```python
from build123d import *

# Parameters (mm, degrees)
SKETCH1_W      = 22
SKETCH1_H      = 12
EXTRUDE1_DEPTH = 10
SKETCH2_W      = 30
SKETCH2_H      = 12
EXTRUDE2_DEPTH = 2
SKETCH3_W      = 22
SKETCH3_H      = 12
EXTRUDE3_DEPTH = 4
SKETCH4_R      = 1
EXTRUDE4_DEPTH = 13
EXTRUDE5_DEPTH = 3.8
SKETCH6_R      = 2.25
EXTRUDE6_DEPTH = 4


with BuildPart() as part:
    # Sketch1 → Extrude1 (new body)
    with BuildSketch(Plane.XY):
        Rectangle(SKETCH1_W, SKETCH1_H)
    extrude(amount=EXTRUDE1_DEPTH)

    # Sketch2 → Extrude2 (add)
    with BuildSketch(Plane.XY.offset(10)):
        Rectangle(SKETCH2_W, SKETCH2_H)
    extrude(amount=EXTRUDE2_DEPTH)

    # Sketch3 → Extrude3 (add)
    with BuildSketch(Plane.XY.offset(12)):
        Rectangle(SKETCH3_W, SKETCH3_H)
    extrude(amount=EXTRUDE3_DEPTH)

    # Sketch4 → Extrude4 (cut, through all)
    with BuildSketch(Plane.XY.offset(12)):
        with Locations((-13, 0)):
            Circle(SKETCH4_R)
        with Locations((13, 0)):
            Circle(SKETCH4_R)
    extrude(amount=-EXTRUDE4_DEPTH, mode=Mode.SUBTRACT)

    # Sketch5 → Extrude5 (add)
    with BuildSketch(Plane.XY.offset(16)):
        with BuildLine():
            ThreePointArc((-0.479166667, -2.445144707), (11, 0), (-0.479166667, 2.445144707))
            ThreePointArc((-0.479166667, 2.445144707), (-3.5, 0), (-0.479166667, -2.445144707))
        make_face()
    extrude(amount=EXTRUDE5_DEPTH)

    # Sketch6 → Extrude6 (add)
    with BuildSketch(Plane.XY.offset(19.8)):
        with Locations((5, 0)):
            Circle(SKETCH6_R)
    extrude(amount=EXTRUDE6_DEPTH)


solid = part.part
```
CAD build for the part. Positions are in the model's coordinates, mm. A direction names the side the tool comes from. Give positions to 0.01 mm unless a question says otherwise; leave off trailing zeros. Order: outer loops, then holes, each group sorted by start corner. A loop starts at its lowest first (then second) coordinate and runs counter-clockwise, first axis right, second up.
(1) Saw through at B-B, the plane x = -1. Give the cut face in (y, z).
(2) Flat gauge pins, fed straight in: pin 1 (2.5 mm diameter, centred on x = 13, y = 0, fed in from +Z); pin 2 (5 mm diameter, centred on y = 0.5, z = 6.5, fed in from -X); pin 3 (1.2 mm diameter, centred on x = -12, y = 1, fed in from -Z); pin 4 (1.2 mm diameter, centred on x = -13, y = 0, fed in from -Z). Where does each tip first touch, or does it go through?
(3) Saw through at C-C, the plane z = 20.75. Give the cut face in (x, y).
(4) Mould opens along X. For faces 5 (the cylindrical face through (7.146, 0.676, 21.772)), 6 (the cylindrical face through (-12, 0, 11)), 7 (the flat face through (11, 0, 5)), 8 (the flat face through (10, 5, 16)) say: released by +X, released by -X, zero draft, split by the parting line, or undercut.
(5) Drill centre lines: L1, parallel to Y at x = -13, z = 11.1; L2, parallel to X at y = 5, z = 13.25; L3, parallel to Z at x = -2.5, y = -3.25. Where is each one in solid material? Low to high.
(6) Saw through at A-A, the plane x = 13. Give the cut face in (y, z).
(7) Saw through at D-D, the plane y = -3. Give the cut face in (x, z).
(8) Tool access for faces 1 (the flat face through (-11.7, 0.1, 12)), 2 (the flat face through (10, -5, 16)), 3 (the flat face through (14.3, 0.1, 10)), 4 (the flat face through (-11.7, 0.1, 10)): list every direction of +Z, -Z, +X, -X, +Y, -Y with a clear straight run to the whole face (end or side of a thin tool).
Results found:
1. outline: (-6, 0) - (6, 0) - (6, 16) - (2.5, 16) - (2.5, 19.8) - (-2.5, 19.8) - (-2.5, 16) - (-6, 16) - close
2. pin 1: stops at z = 12
2. pin 2: stops at x = -11
2. pin 3: stops at z = 10
2. pin 4: passes through
3. outline: circle Ø4.5 at (5, 0)
4. face 5: split by the parting line
4. face 6: undercut
4. face 7: released by +X
4. face 8: zero draft
5. L1: y = -6 to -1, 1 to 6
5. L2: x = -11 to 11
5. L3: z = 0 to 16
6. outline: (-6, 10) - (-1, 10) - (-1, 12) - (-6, 12) - close; (1, 10) - (6, 10) - (6, 12) - (1, 12) - close
7. outline: (-15, 10) - (-11, 10) - (-11, 0) - (11, 0) - (11, 10) - (15, 10) - (15, 12) - (11, 12) - (11, 16) - (10.2, 16) - (10.2, 19.8) - (-0.2, 19.8) - (-0.2, 16) - (-11, 16) - (-11, 12) - (-15, 12) - close
8. face 1: +Z, -X, +Y, -Y
8. face 2: +Z, +X, -Y
8. face 3: -Z, +X, +Y, -Y
8. face 4: -Z, -X, +Y, -Y
